Build history of the part. All positions in model axes, mm. Face numbers are marked on the shaded views. A direction names the side the tool comes from. Round coordinates to 2 decimals unless told otherwise and drop trailing zeros. Write each loop counter-clockwise with the first axis right and the second up, starting at its lowest first coordinate (ties: lowest second). Pieces come first, ordered by that corner, then holes. Notation, with made-up numbers: (75, 89) - (120, 89) arc R13 cw to (120, 98) - close; hole circle Ø4 at (73.25, 27). An arc over 180 degrees is marked (long way). Write each question's results on one line, items separated by ' | '.
from build123d import *

# Parameters (mm, degrees)
SKETCH_1_R          = 9
SKETCH_1_R_2        = 6
EXTRUDE_1_DEPTH     = 40
SKETCH_2_R          = 6.5
CUT_EXTRUDE_1_DEPTH = 5
SKETCH_3_R          = 6.5
CUT_EXTRUDE_2_DEPTH = 5
SKETCH_4_R          = 10
SKETCH_4_R_2        = 9
EXTRUDE_2_DEPTH     = 4


with BuildPart() as part:
    # 草图1 → 凸台-拉伸1 (new body)
    with BuildSketch(Plane.XY):
        Circle(SKETCH_1_R)
        Circle(SKETCH_1_R_2, mode=Mode.SUBTRACT)
    extrude(amount=EXTRUDE_1_DEPTH)

    # 草图2 → 切除-拉伸1 (cut)
    with BuildSketch(Plane.XY.offset(40)):
        Circle(SKETCH_2_R)
    extrude(amount=-CUT_EXTRUDE_1_DEPTH, mode=Mode.SUBTRACT)

    # 草图3 → 切除-拉伸2 (cut)
    with BuildSketch(Plane(origin=(0, 0, 0), x_dir=(-1, 0, 0), z_dir=(0, 0, -1))):
        Circle(SKETCH_3_R)
    extrude(amount=-CUT_EXTRUDE_2_DEPTH, mode=Mode.SUBTRACT)

    # 草图4 → 凸台-拉伸2 (add)
    with BuildSketch(Plane(origin=(0, 0, 0), x_dir=(-1, 0, 0), z_dir=(0, 0, -1))):
        Circle(SKETCH_4_R)
        Circle(SKETCH_4_R_2, mode=Mode.SUBTRACT)
    extrude(amount=-EXTRUDE_2_DEPTH)


solid = part.part
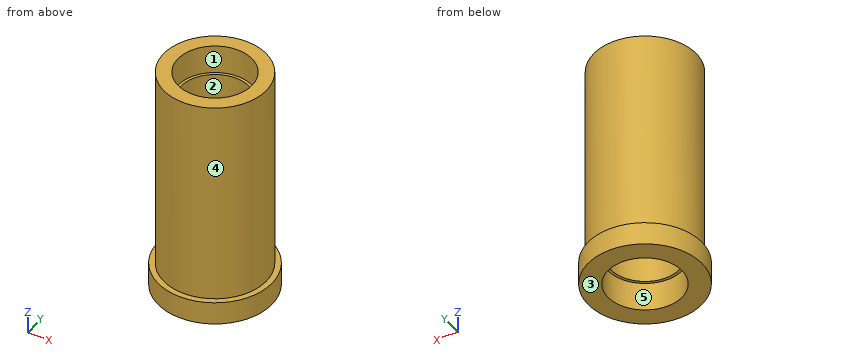
(1) Drill centre lines: probe 1 along Y at (x, z) = (0, 1.7); probe 2 along X at (y, z) = (0, 21.5). Where is each one in solid material? Low to high. Write a range as [from, to].
Worked answers:
probe 1: y = [-10, -6.5], [6.5, 10] | probe 2: x = [-9, -6], [6, 9]
(2) Two-plate mould, pull along Y, no slides. Class the marked faces 3, 4 and 5: released by +Y, released by -Y, zero draft, split by the parting line, or undercut.
Worked answers:
face 3: zero draft | face 4: split by the parting line | face 5: undercut
(3) Slice it at D-D, the plane y = 7.25. Write the cut outline in (x, z), and give its area (3 significant figures).
Worked answers:
outline: (-6.89, 0) - (6.89, 0) - (6.89, 4) - (5.33, 4) - (5.33, 40) - (-5.33, 40) - (-5.33, 4) - (-6.89, 4) - close | area: 439 mm2
(4) Flat gauge pins, fed straight in: pin 1 Ø10.5 at (x, y) = (0, -2) entering from +Z; pin 2 Ø6 at (x, y) = (-2.5, 2) entering from +Z; pin 3 Ø1.5 at (x, z) = (-1, 20.5) entering from -Y; pin 4 Ø11 at (x, y) = (0, 0) entering from +Z. Where does each tip first touch, or does it go through?
Worked answers:
pin 1: stops at z = 40 | pin 2: stops at z = 35 | pin 3: stops at y = -9 | pin 4: passes through
(5) Slice it at A-A, the plane y = 0. Write the cut outline in (x, z), and give its area (3 significant figures).
Worked answers:
outline: (-10, 0) - (-6.5, 0) - (-6.5, 5) - (-6, 5) - (-6, 35) - (-6.5, 35) - (-6.5, 40) - (-9, 40) - (-9, 4) - (-10, 4) - close; (6, 5) - (6.5, 5) - (6.5, 0) - (10, 0) - (10, 4) - (9, 4) - (9, 40) - (6.5, 40) - (6.5, 35) - (6, 35) - close | area: 238 mm2
(6) Tool access for the marked faces 1 and 2: list every direction of +Z, -Z, +X, -X, +Y, -Y with a clear straight run to the whole face (end or side of a thin tool).
Worked answers:
face 1: +Z | face 2: +Z, -Z
(7) Slice it at C-C, the plane z = 3. Write the cut outline in (x, y), and give its area (3 significant figures).
Worked answers:
outline: circle Ø20 at (0, 0); hole circle Ø13 at (0, 0) | area: 181 mm2
